Autodesk Inventor part; units mm, degrees
ref_plane "YZ Plane" through (0, 0, 0) normal (1, 0, 0) x (0, 1, 0)
ref_plane "XZ Plane" through (0, 0, 0) normal (0, 1, 0) x (-1, 0, 0)
ref_plane "XY Plane" through (0, 0, 0) normal (0, 0, 1) x (1, 0, 0)
sketch "Sketch1" plane through (0, 0, 0) normal (0, 1, 0) x (-1, 0, 0)
  line L0 (0, 0) -> (0, -175)
  line L1 (0, -175) -> (6.35, -175)
  line L2 (6.35, -175) -> (6.35, 0)
  line L3 (6.35, 0) -> (0, 0)
  dimension "d0" = 175
  dimension "d1" = 6.35
extrude "Extrusion1" add sketch "Sketch1" along normal blind 6.35
sketch "Sketch2" plane through (0, 6.35, 0) normal (0, 1, 0) x (1, 0, 0)
  line L0 (-6.35, 0) -> (0, 0)
  line L1 (0, 0) -> (-6.35, 17.4465)
  line L2 (-6.35, 175) -> (-6.35, 0)
  line L3 (0, 0) -> (18.5662, 0) construction
  dimension "d4" = 110
extrude "Extrusion2" cut sketch "Sketch2" against normal blind 6.35
sketch "Sketch3" plane through (0, 6.35, 0) normal (0, 1, 0) x (1, 0, 0)
  line L0 (0, 0) -> (0, 175)
  line L1 (0, 175) -> (-6.35, 157.5535)
  line L2 (-6.35, 175) -> (-6.35, 17.4465)
  line L3 (0, 175) -> (18.5662, 175) construction
  line L4 (0, 175) -> (-6.35, 175)
  line L5 (-6.35, 157.5535) -> (-6.35, 175)
  line L6 (-6.35, 175) -> (0, 175)
  dimension "d7" = 110
extrude "Extrusion3" cut sketch "Sketch3" against normal blind 10
properties part number "Top"
Geometry: final body of the model. Coordinates: model frame, mm. Round coordinates to 2 decimals unless told otherwise and drop trailing zeros. Loops run counter-clockwise (first coordinate to the right, second up) from the corner with the lowest first, then second, coordinate; pieces in that order, holes last. Notation, with made-up numbers: M 24.25,63 L 82.25,63 A16 cw 82.25,67 Z; hole C -20,1.5 d1. An arc over 180 degrees is marked long. Put each result on its own line as item: value. Start each with the question number.
(1) Material intervals for line 1 along X through (y, z) = (2.75, -168); line 2 along X through (y, z) = (3, -12.5), sorted ascending. Write a range as [from, to].
(2) Contact query for a flat-ended pin moving along its axis: pin 1 Ø1 at (y, z) = (2.5, -48) entering from +X. Output: stop coordinate, or through.
(3) Section query B-B (x = -2.75). Return loops of the section in (y, z), then the cut area to 3 significant figures.
(4) Section query A-A (y = 4). Return loops of the section in (x, z), then the cut area to 3 significant figures.
Findings below:
1. line 1: x = [-2.55, 0]
1. line 2: x = [-4.55, 0]
2. pin 1: stops at x = 0
3. outline: M 0,-167.44 L 6.35,-167.44 L 6.35,-7.56 L 0,-7.56 Z
3. area: 1,020 mm2
4. outline: M -6.35,-157.55 L 0,-175 L 0,0 L -6.35,-17.45 Z
4. area: 1,000 mm2
